Input: part model. Units: mm. Frame: model coordinates. Face numbers are marked on the shaded views. A direction names the side the tool comes from. Give positions to 0.01 mm unless a question says otherwise; leave off trailing zeros. Write each loop counter-clockwise with the first axis right and the second up, starting at its lowest first coordinate (ties: lowest second). Pieces come first, ordered by that corner, then holes. Notation, with made-up numbers: (24, 80) - (35, 80) arc R14 cw to (35, 95) - close; hole circle Ø4 at (19.5, 57.25). An arc over 180 degrees is marked (long way). Use a Markdown table: item, result. Add a question column.
1. Mould query, pull axis Z, two halves, no side actions, for the marked faces 1, 2 and 3. Classes: released by +Z, released by -Z, zero draft, split by the parting line, or undercut.
2. Set-up query: the marked faces 4 and 5. Return all of +Z, -Z, +X, -X, +Y, -Y with unobstructed straight access to the full face (end or side cutting, diameter ignored); none if empty.
3. Section query A-A, the plane x = 15. Return loops of the section in (y, z) (3 decimals), plus the area to 3 significant figures.
4. Section query C-C, the plane y = -1.5. Return loops of the section in (x, z) (3 decimals).
5. Pin query (flat end, axial travel): pin 1 (4.5 mm diameter, centred on x = 14, z = 7.5, fed in from -Y) (3 decimals); pin 2 (6.5 mm diameter, centred on x = 19, y = -9.5, fed in from -Z). Return the tip coordinate at first contact, or that it passes through.
6. Section query B-B, the plane z = 19.15. Return loops of the section in (x, y) (3 decimals).
7. Material intervals for probe 1 along Z at (x, y) = (36.5, -8.5); probe 2 along Z at (x, y) = (7, -3); probe 3 along X at (y, z) = (-11, 10.75), sorted ascending.
8. Section query D-D, the plane x = 36.5. Return loops of the section in (y, z), plus the area to 3 significant figures.
```python
from build123d import *

# Parameters (mm, degrees)
F0_W     = 42
F0_H     = 24
F1_DEPTH = 15
F2_R     = 2
F3_DEPTH = 25
F4_R     = 4.875
F5_DEPTH = 10.3
F6_R     = 4.875
F7_DEPTH = 13.7
F9_DEPTH = 25


with BuildPart() as f1:
    # F0 (on Front) → F1 (new body)
    with BuildSketch(Plane.XZ):
        with Locations((21, 12)):
            Rectangle(F0_W, F0_H)
    extrude(amount=F1_DEPTH)

    # F2 (on face) → F3 (cut)
    with BuildSketch(Plane.XZ.offset(15)):
        with Locations((5.5, 19.15)):
            Circle(F2_R)
        with Locations((36.5, 19.15)):
            Circle(F2_R)
    extrude(amount=-F3_DEPTH, mode=Mode.SUBTRACT)

    # F4 (on face) → F5 (cut)
    with BuildSketch(Plane.XY.offset(24)):
        with Locations((15, -10)):
            Circle(F4_R)
    extrude(amount=-F5_DEPTH, mode=Mode.SUBTRACT)

    # F6 (on face) → F7 (cut, through all)
    with BuildSketch(Plane(origin=(0, 0, 0), x_dir=(1, 0, 0), z_dir=(0, 0, -1))):
        Polygon((20.9178402592, 15), (9.0821597408, 15), (6.1954083949, 10), (10.5977041974, 2.375), (19.4022958026, 2.375), (23.8045916051, 10), align=None)
        with Locations((15, 10)):
            Circle(F6_R, mode=Mode.SUBTRACT)
        with Locations((15, 10)):
            Circle(F6_R)
    extrude(amount=-F7_DEPTH, mode=Mode.SUBTRACT)

    # F8 (on face) → F9 (cut)
    with BuildSketch(Plane.XZ.offset(15)):
        with BuildLine():
            ThreePointArc((6.1954083949, 7.2318827736), (5.4254083949, 5.85), (6.1954083949, 4.4681172264))
            Line((6.1954083949, 4.4681172264), (6.1954083949, 7.2318827736))
        make_face()
        with BuildLine():
            ThreePointArc((8.5504083949, 6.475), (8.1994569143, 6.9990485194), (7.6754083949, 7.35))
            Line((7.6754083949, 7.35), (6.4254083949, 7.35))
            ThreePointArc((6.4254083949, 7.35), (6.3080554331, 7.2955231165), (6.1954083949, 7.2318827736))
            Line((6.1954083949, 7.2318827736), (6.1954083949, 4.4681172264))
            ThreePointArc((6.1954083949, 4.4681172264), (7.5476247796, 4.3029379887), (8.5504083949, 5.225))
            Line((8.5504083949, 5.225), (8.5504083949, 6.475))
        make_face()
        with BuildLine():
            Line((6.4254083949, 7.35), (7.6754083949, 7.35))
            ThreePointArc((7.6754083949, 7.35), (7.0504083949, 7.475), (6.4254083949, 7.35))
        make_face()
        with BuildLine():
            ThreePointArc((8.6754083949, 5.85), (8.6438519929, 6.1686887196), (8.5504083949, 6.475))
            Line((8.5504083949, 6.475), (8.5504083949, 5.225))
            ThreePointArc((8.5504083949, 5.225), (8.6438519929, 5.5313112804), (8.6754083949, 5.85))
        make_face()
        with BuildLine():
            ThreePointArc((21.4504083949, 6.475), (21.3254083949, 5.85), (21.4504083949, 5.225))
            Line((21.4504083949, 5.225), (21.4504083949, 6.475))
        make_face()
        with BuildLine():
            Line((22.3254083949, 7.35), (23.5754083949, 7.35))
            ThreePointArc((23.5754083949, 7.35), (22.9504083949, 7.475), (22.3254083949, 7.35))
        make_face()
        with BuildLine():
            ThreePointArc((24.5754083949, 5.85), (24.3696815745, 6.6413840039), (23.8045916051, 7.2323878049))
            Line((23.8045916051, 7.2323878049), (23.8045916051, 4.4676121951))
            ThreePointArc((23.8045916051, 4.4676121951), (24.3696815745, 5.0586159961), (24.5754083949, 5.85))
        make_face()
        with BuildLine():
            Line((23.8045916051, 4.4676121951), (23.8045916051, 7.2323878049))
            ThreePointArc((23.8045916051, 7.2323878049), (23.6923341994, 7.2957424046), (23.5754083949, 7.35))
            Line((23.5754083949, 7.35), (22.3254083949, 7.35))
            ThreePointArc((22.3254083949, 7.35), (21.8013598754, 6.9990485194), (21.4504083949, 6.475))
            Line((21.4504083949, 6.475), (21.4504083949, 5.225))
            ThreePointArc((21.4504083949, 5.225), (22.4527349043, 4.3030849743), (23.8045916051, 4.4676121951))
        make_face()
    extrude(amount=-F9_DEPTH, mode=Mode.SUBTRACT)


solid = f1.part
```
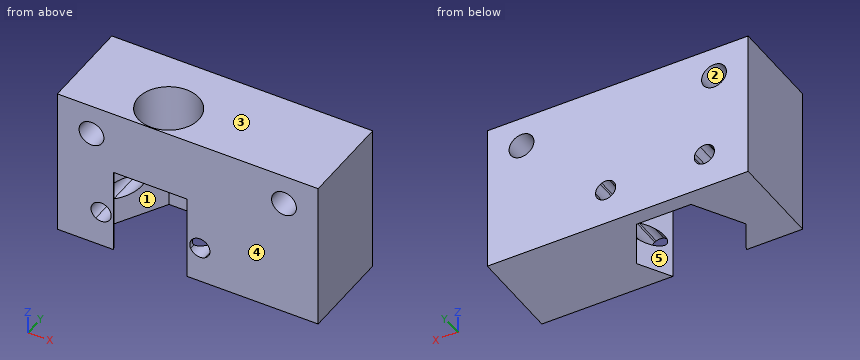
Result sheet:
| question | item | result |
|---|---|---|
| 1 | face 1 | zero draft |
| 1 | face 2 | undercut |
| 1 | face 3 | released by +Z |
| 2 | face 4 | +Z, -Z, +X, -X, -Y |
| 2 | face 5 | -Z |
| 3 | outline | (-15, 13.7) - (-14.875, 13.7) - (-14.875, 24) - (-15, 24) - close; (-5.125, 13.7) - (-2.375, 13.7) - (-2.375, 0) - (0, 0) - (0, 24) - (-5.125, 24) - close |
| 3 | area | 86.6 mm² |
| 4 | outline | (0, 0) - (42, 0) - (42, 24) - (0, 24) - close; hole circle Ø4 at (5.5, 19.15); hole circle Ø3.25 at (7.05, 5.85); hole circle Ø3.25 at (22.95, 5.85); hole circle Ø4 at (36.5, 19.15) |
| 5 | pin 1 | stops at y = -2.375 |
| 5 | pin 2 | stops at z = 13.7 |
| 6 | outline | (0, -15) - (3.5, -15) - (3.5, 0) - (0, 0) - close; (7.5, -15) - (34.5, -15) - (34.5, 0) - (7.5, 0) - close; (38.5, -15) - (42, -15) - (42, 0) - (38.5, 0) - close; hole circle Ø9.75 at (15, -10) |
| 7 | probe 1 | z = 0 to 17.15, 21.15 to 24 |
| 7 | probe 2 | z = 0 to 4.23, 7.47 to 17.83, 20.47 to 24 |
| 7 | probe 3 | x = 0 to 6.77, 23.23 to 42 |
| 8 | outline | (-15, 0) - (0, 0) - (0, 17.15) - (-15, 17.15) - close; (-15, 21.15) - (0, 21.15) - (0, 24) - (-15, 24) - close |
| 8 | area | 300 mm² |
